from build123d import *

# Parameters (mm, degrees)
F0_R     = 11.1
F1_DEPTH = 20
F2_R     = 5.125
F3_DEPTH = 6
F4_SIZE  = 2
F5_SIZE  = 0.5


with BuildPart() as f1:
    # F0 (on Front) → F1 (new body)
    with BuildSketch(Plane.XZ):
        Circle(F0_R)
    extrude(amount=F1_DEPTH)

    # F2 (on face) → F3 (join)
    with BuildSketch(Plane.XZ.offset(20)):
        Circle(F2_R)
    extrude(amount=F3_DEPTH)

    # F4
    f4_edges = [f1.edges().sort_by_distance(p)[0] for p in [
        (-5.125, -26, 0),
    ]]
    chamfer(f4_edges, length=F4_SIZE)

    # F5
    f5_edges = [f1.edges().sort_by_distance(p)[0] for p in [
        (-11.1, -20, 0),
    ]]
    chamfer(f5_edges, length=F5_SIZE)


solid = f1.part
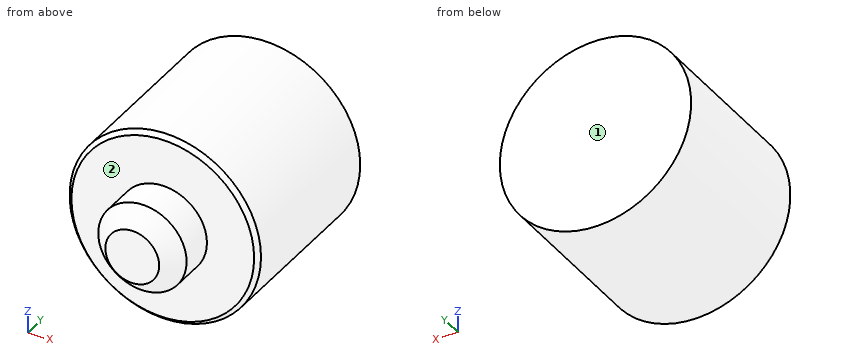
Can you work these out from the model? Positions are in its coordinate system, mm. Face numbers are marked on the shaded views. A direction names the side the tool comes from. Round coordinates to 2 decimals unless told otherwise and drop trailing zeros. Write each loop counter-clockwise with the first axis right and the second up, starting at its lowest first coordinate (ties: lowest second). Pieces come first, ordered by that corner, then holes. Notation, with made-up numbers: (8.25, 56.5) - (42.25, 56.5) arc R20 ccw to (42.25, 63.5) - close; hole circle Ø1 at (-14, 72.25). An arc over 180 degrees is marked (long way). Write each question's results on one line, items separated by ' | '. Start each with the question number.
1) Suppose I cut it at A-A (z = 0). List the corners of the cut face in (x, y) for me (3 decimals), and give its area (3 significant figures).
2) Suppose I cut it at C-C (y = -8). List the corners of the cut face in (x, z) for me.
3) Which directions (+Z, -Z, +X, -X, +Y, -Y) give clear straight access to the entire face, cutting with the end or side of a thin tool? Please do the marked faces 1 and 2.
4) Suppose I cut it at B-B (x = 0). List the corners of the cut face in (y, z) for me (3 decimals), and give its area (3 significant figures).
5) For pin 1 Ø2 at (x, y) = (-2, -19.5) entering from +Z; pin 2 Ø1.5 at (y, z) = (-21, 5) entering from -X; pin 3 Ø6 at (x, y) = (5.5, -20) entering from +Z (3 decimals), each with a flat end and sliding along its axis, tell me the tip position at first contact or that it passes through.
6) Please list where these lines run through material, in increasing order: line 1 (Y direction, x = 3.25, z = -6.5); line 2 (X direction, y = -21.5, z = 0.25); line 3 (X direction, y = -4, z = -4).
Here are the results:
1) outline: (-11.1, -19.5) - (-10.6, -20) - (-5.125, -20) - (-5.125, -24) - (-3.125, -26) - (3.125, -26) - (5.125, -24) - (5.125, -20) - (10.6, -20) - (11.1, -19.5) - (11.1, 0) - (-11.1, 0) - close | area: 501 mm2
2) outline: circle Ø22.2 at (0, 0)
3) face 1: +Z, -Z, +X, -X, +Y | face 2: -Y
4) outline: (-26, -3.125) - (-24, -5.125) - (-20, -5.125) - (-20, -10.6) - (-19.5, -11.1) - (0, -11.1) - (0, 11.1) - (-19.5, 11.1) - (-20, 10.6) - (-20, 5.125) - (-24, 5.125) - (-26, 3.125) - close | area: 501 mm2
5) pin 1: stops at z = 11.05 | pin 2: stops at x = -2.86 | pin 3: stops at z = 10.805
6) line 1: y = -20 to 0 | line 2: x = -5.12 to 5.12 | line 3: x = -10.35 to 10.35
